Work out the finished part from the listing and answer in its coordinate system (mm). Face numbers are marked on the shaded views. A direction names the side the tool comes from. Round coordinates to 2 decimals unless told otherwise and drop trailing zeros. Order: outer loops, then holes, each group sorted by start corner. A loop starts at its lowest first (then second) coordinate and runs counter-clockwise, first axis right, second up. Notation, with made-up numbers: (43, 84) - (90, 84) arc R18 ccw to (90, 93) - close; hole circle Ø2 at (48, -31). An arc over 180 degrees is marked (long way). Use one line per item in the form item = value. Start each with the question number.
Q1. The part is cut by section D-D on y = 7.5. Determine the outline of the cut face in (x, z).
Q2. The part is cut by section B-B on x = 0. Determine the outline of the cut face in (y, z).
Q3. The part is cut by section C-C on y = -2. Determine the outline of the cut face in (x, z), plus the area to 3 significant figures.
Q4. Find the intervals of material crossed by line 1 (X direction, y = -3.5, z = 0); line 2 (Z direction, x = 0, y = 16.5); line 3 (Z direction, x = 3, y = -3), in increasing order. Write a range as [from, to].
Q5. Given P1, Ø3, axis at x = -17, y = 15.5, coming from the -Z side; P2, Ø10, axis at x = 0, y = 31.75, coming from the +Z side; P3, Ø1.5, axis at x = -6, y = 2.5, coming from the +Z side, each flat-ended and moving along its own axis, determine where each tip first touches the part or whether it passes through.
Q6. For a pull along Z with two mould halves and no side action, classify the marked faces 1, 2 and 3 as +Z half, -Z half, draft (parallel to the pull), parting line (faces both ways), or undercut.
Q7. The part is cut by section A-A on z = 0. Determine the outline of the cut face in (x, y), plus the area to 3 significant figures.
Q8. Which of the six approach directions +Z, -Z, +X, -X, +Y, -Y give full straight-line access (tool end or side, diameter ignored) to the marked faces 4, 5 and 6?
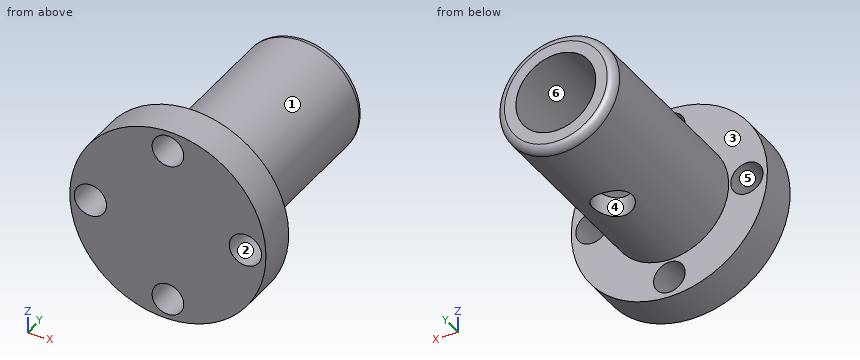
from build123d import *

# Parameters (mm, degrees)
SKETCH1_R                                  = 19.05
BOSS_EXTRUDE1_DEPTH                        = 63.5
SKETCH2_R                                  = 12.826740919
CUT_EXTRUDE1_DEPTH                         = 69.978656119
SKETCH3_R                                  = 6.33257482
CUT_EXTRUDE2_DEPTH                         = 69.978656119
FILLET1_R                                  = 2.54
SKETCH4_R                                  = 31.496
BOSS_EXTRUDE3_DEPTH                        = 12.7
SKETCH5_R                                  = 5.075123318
CUT_EXTRUDE3_DEPTH                         = 78.564463801
MIRROR1_AT_THE_SECOND_PLANE_COPY_1_SKETC_R = 5.075123318
MIRROR1_AT_THE_SECOND_PLANE_COPY_1_DEPTH   = 78.564463801
SKETCH6_R                                  = 5.182943359
CUT_EXTRUDE4_DEPTH                         = 78.564463801
MIRROR2_AT_THE_SECOND_PLANE_COPY_1_SKETC_R = 5.182943359
MIRROR2_AT_THE_SECOND_PLANE_COPY_1_DEPTH   = 78.564463801


with BuildPart() as part:
    # Sketch1 → Boss-Extrude1 (new body)
    with BuildSketch(Plane(origin=(0, 0, 0), x_dir=(1, 0, 0), z_dir=(0, 1, 0))):
        with Locations(Location((0, 0, 0), (0, 0, 270))):
            Circle(SKETCH1_R)
    extrude(amount=BOSS_EXTRUDE1_DEPTH)

    # Sketch2 → Cut-Extrude1 (cut, through all)
    with BuildSketch(Plane(origin=(0, 63.5, 0), x_dir=(1, 0, 0), z_dir=(0, 1, 0))):
        with Locations(Location((0, 0, 0), (0, 0, 270))):
            Circle(SKETCH2_R)
    extrude(amount=-CUT_EXTRUDE1_DEPTH, mode=Mode.SUBTRACT)

    # Sketch3 → Cut-Extrude2 (cut, through all)
    with BuildSketch(Plane.XY):
        with Locations((0, 31.75)):
            Circle(SKETCH3_R)
    extrude(amount=-CUT_EXTRUDE2_DEPTH, mode=Mode.SUBTRACT)

    # Fillet1
    fillet1_edges = [part.edges().sort_by_distance(p)[0] for p in [
        (0, 63.5, -19.05),
    ]]
    fillet(fillet1_edges, radius=FILLET1_R)

    # Sketch4 → Boss-Extrude3 (add)
    with BuildSketch(Plane.XZ):
        with Locations(Location((0, 0, 0), (0, 0, 270))):
            Circle(SKETCH4_R)
    extrude(amount=BOSS_EXTRUDE3_DEPTH)

    # Sketch5 → Cut-Extrude3 (cut, through all)
    with BuildSketch(Plane(origin=(0, 0, 0), x_dir=(1, 0, 0), z_dir=(0, 1, 0))):
        with Locations(Location((0, 24.892, 0), (0, 0, 270))):
            Circle(SKETCH5_R)
    cut_extrude3 = extrude(amount=-CUT_EXTRUDE3_DEPTH, mode=Mode.SUBTRACT)

    # Mirror1: Cut-Extrude3 across plane
    add(cut_extrude3.mirror(Plane(origin=(0, 0, 0), x_dir=(0, 0, 1), z_dir=(1, 0, 0))), mode=Mode.SUBTRACT)

    # Mirror1 at the second plane: Cut-Extrude3 across plane
    add(cut_extrude3.mirror(Plane.XY), mode=Mode.SUBTRACT)

    # Mirror1 at the second plane copy 1 sketc → Mirror1 at the second plane copy 1 (cut, through all)
    with BuildSketch(Plane(origin=(0, 0, 0), x_dir=(-1, 0, 0), z_dir=(0, 1, 0))):
        with Locations(Location((0, 24.892, 0), (0, 0, 270))):
            Circle(MIRROR1_AT_THE_SECOND_PLANE_COPY_1_SKETC_R)
    extrude(amount=-MIRROR1_AT_THE_SECOND_PLANE_COPY_1_DEPTH, mode=Mode.SUBTRACT)

    # Sketch6 → Cut-Extrude4 (cut, through all)
    with BuildSketch(Plane(origin=(0, 0, 0), x_dir=(1, 0, 0), z_dir=(0, 1, 0))):
        with Locations(Location((24.892, 0, 0), (0, 0, 270))):
            Circle(SKETCH6_R)
    cut_extrude4 = extrude(amount=-CUT_EXTRUDE4_DEPTH, mode=Mode.SUBTRACT)

    # Mirror2: Cut-Extrude4 across plane
    add(cut_extrude4.mirror(Plane.XY), mode=Mode.SUBTRACT)

    # Mirror2 at the second plane: Cut-Extrude4 across plane
    add(cut_extrude4.mirror(Plane(origin=(0, 0, 0), x_dir=(0, 0, 1), z_dir=(1, 0, 0))), mode=Mode.SUBTRACT)

    # Mirror2 at the second plane copy 1 sketc → Mirror2 at the second plane copy 1 (cut, through all)
    with BuildSketch(Plane(origin=(0, 0, 0), x_dir=(-1, 0, 0), z_dir=(0, 1, 0))):
        with Locations(Location((24.892, 0, 0), (0, 0, 270))):
            Circle(MIRROR2_AT_THE_SECOND_PLANE_COPY_1_SKETC_R)
    extrude(amount=-MIRROR2_AT_THE_SECOND_PLANE_COPY_1_DEPTH, mode=Mode.SUBTRACT)


solid = part.part
Found:
q1.outline = circle Ø38.1 at (0, 0); hole circle Ø25.65 at (0, 0)
q2.outline = (-12.7, -31.5) - (0, -31.5) - (0, -29.97) - (-12.7, -29.97) - close; (-12.7, -19.82) - (0, -19.82) - (0, -19.05) - (25.42, -19.05) - (25.42, -12.83) - (0, -12.83) - (0, 12.83) - (63.5, 12.83) - (63.5, 16.51) arc R2.54 ccw to (60.96, 19.05) - (0, 19.05) - (0, 19.82) - (-12.7, 19.82) - close; (-12.7, 29.97) - (0, 29.97) - (0, 31.5) - (-12.7, 31.5) - close; (38.08, -19.05) - (60.96, -19.05) arc R2.54 ccw to (63.5, -16.51) - (63.5, -12.83) - (38.08, -12.83) - close
q3.outline = circle Ø62.99 at (0, 0); hole circle Ø10.37 at (-24.89, 0); hole circle Ø10.15 at (0, -24.89); hole circle Ø10.15 at (0, 24.89); hole circle Ø10.37 at (24.89, 0)
q3.area = 2,790 mm²
q4.line_1 = [-31.5, -30.07], [-19.71, 19.71], [30.07, 31.5]
q4.line_2 = [-19.05, -12.83], [12.83, 19.05]
q4.line_3 = [-31.35, -28.99], [-20.8, 20.8], [28.99, 31.35]
q5.P1 = -11.07
q5.P2 = 19.05
q5.P3 = 18.31
q6.face_1 = parting line
q6.face_2 = undercut
q6.face_3 = draft
q7.outline = (-31.5, -12.7) - (-30.07, -12.7) - (-30.07, 0) - (-31.5, 0) - close; (-19.71, -12.7) - (19.71, -12.7) - (19.71, 0) - (19.05, 0) - (19.05, 60.96) arc R2.54 ccw to (16.51, 63.5) - (12.83, 63.5) - (12.83, 0) - (-12.83, 0) - (-12.83, 63.5) - (-16.51, 63.5) arc R2.54 ccw to (-19.05, 60.96) - (-19.05, 0) - (-19.71, 0) - close; (30.07, -12.7) - (31.5, -12.7) - (31.5, 0) - (30.07, 0) - close
q7.area = 1,320 mm²
q8.face_4 = -Z
q8.face_5 = +Y, -Y
q8.face_6 = +Y
